```python
from build123d import *

# Parameters (mm, degrees)
F0_W        = 122.399628
F0_H        = 78.418762
F1_DEPTH    = 50.8
F2_R        = 9.36089
F2_R_2      = 8.424406
F3_DEPTH    = 101.6
F3_FACE_R   = 9.36089
F3_FACE_R_2 = 8.424406
F4_DEPTH    = 101.6


with BuildPart() as f1:
    # F0 (on Top) → F1 (new body)
    with BuildSketch(Plane.XY):
        Rectangle(F0_W, F0_H)
    extrude(amount=F1_DEPTH)

    # F2 (on Top) → F3 (join)
    with BuildSketch(Plane.XY):
        with Locations((-37.34231, 0)):
            Circle(F2_R)
        with Locations((37.549719, 0)):
            Circle(F2_R_2)
    extrude(amount=F3_DEPTH)

    # F3_face (on face) → F4 (cut)
    with BuildSketch(Plane(origin=(-37.34231, 0, 101.6), x_dir=(1, 0, 0), z_dir=(0, 0, 1))):
        Circle(F3_FACE_R)
        with Locations((74.892029, 0)):
            Circle(F3_FACE_R_2)
    extrude(amount=-F4_DEPTH, mode=Mode.SUBTRACT)


solid = f1.part
```
For this review, take the finished solid that the model builds, in its own axes (mm). Coordinates: 2 decimals unless noted, no trailing zeros. Write each loop counter-clockwise with the first axis right and the second up, starting at its lowest first coordinate (ties: lowest second). Pieces come first, ordered by that corner, then holes.
(1) Wall thickness on probe 1 along X at (y, z) = (0, 22.5); probe 2 along Y at (x, z) = (-37.5, 35); probe 3 along Y at (x, z) = (-39, 19): over which ranges is each line inside the solid? List them lowest first.
(2) The part is to be moulded in two halves that separate along X. For faces 1 (the face through (-1, 39.209, 25)), 2 (the face through (45.585, 2.53, 25.756)), 3 (the face through (61.2, -1, 25)), 4 (the face through (-28.414, 2.812, 25.756)), say which applies: +X half, -X half, draft (parallel to the pull), parting line (faces both ways), or undercut.
(3) For pin 1 Ø17 at (x, y) = (-37.34, 0) entering from +Z, flat-tipped, find the tip position at first contact; note if it passes through.
(4) Add section B-B on z = 12. Give the boundary of the cut face in (x, y), then the cut area to 3 significant figures.
(5) Add section A-A on y = 0. Give the boundary of the cut face in (x, z).
(6) Add section C-C on x = -38. Give the boundary of the cut face in (y, z), then the cut area to 3 significant figures.
Answer sheet:
1. probe 1: x = -61.2 to -46.7, -27.98 to 29.13, 45.97 to 61.2
1. probe 2: y = -39.21 to -9.36, 9.36 to 39.21
1. probe 3: y = -39.21 to -9.21, 9.21 to 39.21
2. face 1: draft
2. face 2: undercut
2. face 3: +X half
2. face 4: undercut
3. pin 1: passes through
4. outline: (-61.2, -39.21) - (61.2, -39.21) - (61.2, 39.21) - (-61.2, 39.21) - close; hole circle Ø18.72 at (-37.34, 0); hole circle Ø16.85 at (37.55, 0)
4. area: 9,100 mm2
5. outline: (-61.2, 0) - (-46.7, 0) - (-46.7, 50.8) - (-61.2, 50.8) - close; (-27.98, 0) - (29.13, 0) - (29.13, 50.8) - (-27.98, 50.8) - close; (45.97, 0) - (61.2, 0) - (61.2, 50.8) - (45.97, 50.8) - close
6. outline: (-39.21, 0) - (-9.34, 0) - (-9.34, 50.8) - (-39.21, 50.8) - close; (9.34, 0) - (39.21, 0) - (39.21, 50.8) - (9.34, 50.8) - close
6. area: 3,030 mm2
